Model file for the job. Use its own axes, mm. A direction names the side the tool comes from. Round coordinates to 2 decimals unless told otherwise and drop trailing zeros. Order: outer loops, then holes, each group sorted by start corner. A loop starts at its lowest first (then second) coordinate and runs counter-clockwise, first axis right, second up. Notation, with made-up numbers: (14.25, 51) -> (38.25, 51) arc R25 ccw to (38.25, 72) -> close; hole circle Ø2 at (3.5, 51.25). An arc over 180 degrees is marked (long way). Use CSV: the item, a comma, the result in double quotes.
```python
from build123d import *

# Parameters (mm, degrees)
SKETCH1_R           = 25
BOSS_EXTRUDE1_DEPTH = 80
CUT_EXTRUDE1_DEPTH  = 80
SKETCH3_R           = 10
CUT_EXTRUDE2_DEPTH  = 80


with BuildPart() as part:
    # Sketch1 → Boss-Extrude1 (new body)
    with BuildSketch(Plane.XY):
        with BuildLine():
            Line((-107.76864352, 0), (107.76864352, 0))
            Line((107.76864352, 0), (107.76864352, 20))
            Line((107.76864352, 20), (57.5, 20))
            ThreePointArc((57.5, 20), (43.357864376, 25.857864376), (37.5, 40))
            ThreePointArc((37.5, 40), (0, 77.5), (-37.5, 40))
            ThreePointArc((-37.5, 40), (-43.357864376, 25.857864376), (-57.5, 20))
            Line((-57.5, 20), (-107.76864352, 20))
            Line((-107.76864352, 20), (-107.76864352, 0))
        make_face()
        with Locations((0, 40)):
            Circle(SKETCH1_R, mode=Mode.SUBTRACT)
    extrude(amount=-BOSS_EXTRUDE1_DEPTH)

    # Sketch2 → Cut-Extrude1 (cut)
    with BuildSketch(Plane(origin=(0, 20, 0), x_dir=(1, 0, 0), z_dir=(0, 1, 0))):
        with BuildLine():
            Line((-107.76864352, 0), (-67.76864352, 0))
            ThreePointArc((-67.76864352, 0), (-96.052914767, 11.715728753), (-107.76864352, 40))
            Line((-107.76864352, 40), (-107.76864352, 0))
        make_face()
        with BuildLine():
            ThreePointArc((-107.76864352, 40), (-96.052914767, 68.284271247), (-67.76864352, 80))
            Line((-67.76864352, 80), (-107.76864352, 80))
            Line((-107.76864352, 80), (-107.76864352, 40))
        make_face()
        with BuildLine():
            ThreePointArc((107.76864352, 40), (96.052914767, 11.715728753), (67.76864352, 0))
            Line((67.76864352, 0), (107.76864352, 0))
            Line((107.76864352, 0), (107.76864352, 40))
        make_face()
        with BuildLine():
            Line((107.76864352, 80), (67.76864352, 80))
            ThreePointArc((67.76864352, 80), (96.052914767, 68.284271247), (107.76864352, 40))
            Line((107.76864352, 40), (107.76864352, 80))
        make_face()
    extrude(amount=-CUT_EXTRUDE1_DEPTH, mode=Mode.SUBTRACT)

    # Sketch3 → Cut-Extrude2 (cut)
    with BuildSketch(Plane(origin=(0, 20, 0), x_dir=(1, 0, 0), z_dir=(0, 1, 0))):
        with Locations(Location((70, 40, 0), (0, 0, 270))):
            Circle(SKETCH3_R)
        with Locations(Location((-70, 40, 0), (0, 0, 270))):
            Circle(SKETCH3_R)
    extrude(amount=-CUT_EXTRUDE2_DEPTH, mode=Mode.SUBTRACT)


solid = part.part
```
Q1. Pin check, flat tips, straight feed: pin 1 (6 mm diameter, centred on y = 19.5, z = -11.5, fed in from +X); pin 2 (18 mm diameter, centred on x = -70, z = -40, fed in from -Y); pin 3 (6 mm diameter, centred on x = 3, z = -52.5, fed in from +Y); pin 4 (25 mm diameter, centred on x = 81, z = -20.5, fed in from +Y). Stop position of each tip, or through.
From the geometry:
pin 1,"stops at x = 98.59"
pin 2,"passes through"
pin 3,"stops at y = 77.5"
pin 4,"stops at y = 20"
Q2. Which spindle directions (+Z, -Z, +X, -X, +Y, -Y) get a long thin tool onto all of the face, cutting with end or side? Do faces 5 (the flat face through (-1, 13, 0)), 6 (the flat face through (83, 20, -39)). Say none if no direction does.
From the geometry:
face 5,"+Z, +X, -X, +Y, -Y"
face 6,"+Z, -Z, +X, +Y"
Q3. Cut at B-B (z = -46.5). Give the cut face in (x, y).
From the geometry:
outline,"(-107.24, 0) -> (-77.6, 0) -> (-77.6, 20) -> (-107.24, 20) -> close; (-62.4, 0) -> (62.4, 0) -> (62.4, 20) -> (57.5, 20) arc R20 cw to (37.5, 40) arc R37.5 ccw to (-37.5, 40) arc R20 cw to (-57.5, 20) -> (-62.4, 20) -> close; (77.6, 0) -> (107.24, 0) -> (107.24, 20) -> (77.6, 20) -> close; hole circle Ø50 at (0, 40)"
Q4. Cut at A-A (x = 0). Give the cut face in (y, z).
From the geometry:
outline,"(0, -80) -> (15, -80) -> (15, 0) -> (0, 0) -> close; (65, -80) -> (77.5, -80) -> (77.5, 0) -> (65, 0) -> close"
Q5. Cut at C-C (y = 22). Give the cut face in (x, z), plus the area to 3 significant figures.
From the geometry:
outline,"(-48.78, -80) -> (-17.35, -80) -> (-17.35, 0) -> (-48.78, 0) -> close; (17.35, -80) -> (48.78, -80) -> (48.78, 0) -> (17.35, 0) -> close"
area,"5,030 mm²"
Q6. Mould opens along Z. For faces 1 (the flat face through (-1, 13, -80)), 2 (the cylindrical face through (-70, 10, -50)), 3 (the cylindrical face through (79.915, 10.14, -41.302)), 4 (the flat face through (-82, 20, -39)) say: +Z half, -Z half, draft (parallel to the pull), parting line (faces both ways), or undercut.
From the geometry:
face 1,"-Z half"
face 2,"undercut"
face 3,"undercut"
face 4,"draft"
Q7. Cut at D-D (z = -6). Give the cut face in (x, y), plus the area to 3 significant figures.
From the geometry:
outline,"(-88.84, 0) -> (88.84, 0) -> (88.84, 20) -> (57.5, 20) arc R20 cw to (37.5, 40) arc R37.5 ccw to (-37.5, 40) arc R20 cw to (-57.5, 20) -> (-88.84, 20) -> close; hole circle Ø50 at (0, 40)"
area,"5,470 mm²"
Q8. Probe line 1 along X through (y, z) = (14.5, -40); line 2 along Y through (x, z) = (0, -40); line 3 along Y through (x, z) = (65.5, -56). List the from-to ranges inside material, lowest first.
From the geometry:
line 1,"x = -107.77 to -80, -60 to 60, 80 to 107.77"
line 2,"y = 0 to 15, 65 to 77.5"
line 3,"y = 0 to 20"
